from build123d import *

# Parameters (mm, degrees)
SKETCH5_W           = 30
SKETCH5_H           = 30
BOSS_EXTRUDE3_DEPTH = 40
CUT_EXTRUDE1_DEPTH  = 50
SKETCH8_W           = 4.9
SKETCH8_H           = 6
CUT_EXTRUDE3_DEPTH  = 40
SKETCH10_W          = 3
SKETCH10_H          = 40
BOSS_EXTRUDE4_DEPTH = 10
SKETCH11_W          = 37
SKETCH11_H          = 37
BOSS_EXTRUDE5_DEPTH = 50
SKETCH14_R          = 1.5
CUT_EXTRUDE4_DEPTH  = 20
FILLET2_R           = 15
FILLET3_R           = 3
FILLET4_R           = 10
SKETCH15_W          = 3
SKETCH15_H          = 40
BOSS_EXTRUDE6_DEPTH = 10


# Some blends are built 0.0001 mm under size
with BuildPart() as part:
    # Sketch5 → Boss-Extrude3 (new body)
    with BuildSketch(Plane(origin=(0, 0, 0), x_dir=(1, 0, 0), z_dir=(0, 1, 0))):
        with Locations((15, -15)):
            Rectangle(SKETCH5_W, SKETCH5_H)
    extrude(amount=BOSS_EXTRUDE3_DEPTH)

    # Sketch6 → Cut-Extrude1 (cut)
    with BuildSketch(Plane(origin=(0, 40, 0), x_dir=(1, 0, 0), z_dir=(0, 1, 0))):
        Polygon((12.2, -5), (4.9, -5), (4.9, -15.05), (20.1, -15.05), (20.1, -12.3), (23, -10.3), (23, -12.3), (25, -12.3), (25, -5), (17.7, -5), (17.7, -7), (19.7, -7), (17.7, -9.9), (12.2, -9.9), (10.2, -7), (12.2, -7), align=None)
        Polygon((20.1, -15.05), (4.9, -15.05), (4.9, -25.1), (12.2, -25.1), (12.2, -23.1), (10.2, -23.1), (12.2, -20.2), (17.7, -20.2), (19.7, -23.1), (17.7, -23.1), (17.7, -25.1), (25, -25.1), (25, -17.8), (23, -17.8), (23, -19.8), (20.1, -17.8), align=None)
    extrude(amount=-CUT_EXTRUDE1_DEPTH, mode=Mode.SUBTRACT)

    # Sketch8 → Cut-Extrude3 (cut)
    with BuildSketch(Plane(origin=(0, 40, 0), x_dir=(1, 0, 0), z_dir=(0, 1, 0))):
        with Locations((2.45, -15)):
            Rectangle(SKETCH8_W, SKETCH8_H)
    extrude(amount=-CUT_EXTRUDE3_DEPTH, mode=Mode.SUBTRACT)

    # Sketch10 → Boss-Extrude4 (add)
    with BuildSketch(Plane.ZY):
        with Locations((1.5, 20)):
            Rectangle(SKETCH10_W, SKETCH10_H)
        with Locations((10.5, 20)):
            Rectangle(SKETCH10_W, SKETCH10_H)
        with Locations((19.5, 20)):
            Rectangle(SKETCH10_W, SKETCH10_H)
    extrude(amount=BOSS_EXTRUDE4_DEPTH)

    # Sketch11 → Boss-Extrude5 (add)
    with BuildSketch(Plane(origin=(0, 0, 0), x_dir=(-1, 0, 0), z_dir=(0, 0, -1))):
        with Locations((-10, 20)):
            Rectangle(SKETCH11_W, SKETCH11_H)
    extrude(amount=BOSS_EXTRUDE5_DEPTH)

    # Sketch14 → Cut-Extrude4 (cut)
    with BuildSketch(Plane(origin=(0, 0, -50), x_dir=(-1, 0, 0), z_dir=(0, 0, -1))):
        with Locations((-10.1, 32.75)):
            Circle(SKETCH14_R)
        with Locations((1.591342951, 12.5)):
            Circle(SKETCH14_R)
        with Locations((-21.791342951, 12.5)):
            Circle(SKETCH14_R)
    extrude(amount=-CUT_EXTRUDE4_DEPTH, mode=Mode.SUBTRACT)

    # Fillet2
    fillet2_edges = [part.edges().sort_by_distance(p)[0] for p in [
        (28.5, 38.5, -25),
        (28.5, 1.5, -25),
        (-8.5, 1.5, -25),
        (-8.5, 38.5, -25),
    ]]
    fillet(fillet2_edges, radius=FILLET2_R)

    # Fillet3
    fillet3_edges = [part.edges().sort_by_distance(p)[0] for p in [
        (0, 20, 3),
        (0, 20, 9),
    ]]
    fillet(fillet3_edges, radius=FILLET3_R - 0.0001)  # a hair under: the kernel refuses the full size

    # Fillet4
    # the kernel refuses this fillet: 10 mm, written as the material it adds along each edge
    with BuildSketch(Plane(origin=(0, 0, 21), x_dir=(0, 0, 1), z_dir=(0, 1, 0))) as fillet4_piece_1:
        with BuildLine():
            CenterArc((10, -9.949874371), FILLET4_R, 95.739170477, 84.260829523)
            Line((0, -9.949874371), (-0.2, -9.949874371))
            Line((-0.2, -9.949874371), (-0.2, 0))
            Line((-0.2, 0), (0, 0.2))
            ThreePointArc((0, 0.2), (4.5, 0.2), (8.98, 0.198997487))
            Line((8.98, 0.198997487), (9, 0))
        make_face()
    extrude(amount=40)

    # Sketch15 → Boss-Extrude6 (add)
    with BuildSketch(Plane.ZY.offset(10)):
        with Locations((10.5, 20)):
            Rectangle(SKETCH15_W, SKETCH15_H)
        with Locations((19.5, 20)):
            Rectangle(SKETCH15_W, SKETCH15_H)
    extrude(amount=BOSS_EXTRUDE6_DEPTH)


solid = part.part
For this review, take the finished solid that the model builds, in its own axes (mm). A direction names the side the tool comes from. Give positions to 0.01 mm unless a question says otherwise; leave off trailing zeros. Loops run counter-clockwise (first coordinate to the right, second up) from the corner with the lowest first, then second, coordinate; pieces in that order, holes last.
Item 1: Insertion check: pin 1 (11 mm diameter, centred on x = -15.5, y = 21, fed in from +Z); pin 2 (4 mm diameter, centred on y = 22, z = -35, fed in from -X); pin 3 (1.5 mm diameter, centred on x = 10, y = 33, fed in from -Z); pin 4 (12 mm diameter, centred on x = 5.5, z = 11, fed in from +Y). Each pin has a flat end and moves straight along its axis. Give the tip position at first contact, or say it passes through.
Item 2: Take a section at A-A, the plane x = -13. State the section outline as (y, z) points, and give its area (3 significant figures).
Item 3: Take a section at D-D, the plane x = 2. State the section outline as (y, z) points.
Item 4: Draft analysis for pull direction X (two halves, no side actions). For faces 4 (the flat face through (12.2, 20, 6)), 5 (the flat face through (11.186, 20.28, 21.67)), 6 (the flat face through (-10, 20, 1)), 7 (the flat face through (30, 20, 15)), state which applies: +X half, -X half, draft (parallel to the pull), parting line (faces both ways), or undercut.
Item 5: Take a section at C-C, the plane x = 15. State the section outline as (y, z) points.
Item 6: For line 1 along Z through (x, y) = (13.5, 25.5); line 2 along Z through (x, y) = (7.5, 30); line 3 along Y through (x, z) = (10, -41), list the stretches that pass through material, from the lowest coordinate up.
Item 7: Take a section at B-B, the plane z = -9. State the section outline as (x, y) points.
Item 8: Tool access review of faces 1 (the cylindrical face through (-0.86, 20.28, 8.1)), 2 (the cylindrical face through (-1.266, 11.036, -40.14)), 3 (the flat face through (25, 20, 9)): name each direction out of +Z, -Z, +X, -X, +Y, -Y from which nothing blocks a thin tool from reaching the whole face with its end or side.
Calculated:
1. pin 1: stops at z = 21
1. pin 2: stops at x = -8.5
1. pin 3: stops at z = -30
1. pin 4: stops at y = 40
2. outline: (0, 9) - (40, 9) - (40, 12) - (0, 12) - close; (0, 18) - (40, 18) - (40, 21) - (0, 21) - close
2. area: 240 mm2
3. outline: (0, 0) - (2.19, 0) - (2.19, -50) - (37.81, -50) - (37.81, 0) - (40, 0) - (40, 12) - (0, 12) - close; (0, 18) - (40, 18) - (40, 30) - (0, 30) - close
4. face 4: undercut
4. face 5: undercut
4. face 6: -X half
4. face 7: +X half
5. outline: (0, 0) - (1.58, 0) - (1.58, -50) - (38.42, -50) - (38.42, 0) - (40, 0) - (40, 9.9) - (0, 9.9) - close; (0, 20.2) - (40, 20.2) - (40, 30) - (0, 30) - close
6. line 1: z = -50 to 9.9, 20.2 to 30
6. line 2: z = -50 to 5, 25.1 to 30
6. line 3: y = 1.5 to 31.25, 34.25 to 38.5
7. outline: (-8.5, 16.5) arc R15 ccw to (6.5, 1.5) - (13.5, 1.5) arc R15 ccw to (28.5, 16.5) - (28.5, 23.5) arc R15 ccw to (13.5, 38.5) - (6.5, 38.5) arc R15 ccw to (-8.5, 23.5) - close
8. face 1: -X, +Y, -Y
8. face 2: -Z
8. face 3: +Y, -Y
